```python
from build123d import *

# Parameters (mm, degrees)
SKETCH1_W           = 200
SKETCH1_H           = 100
SKETCH1_R           = 2.5
BOSS_EXTRUDE1_DEPTH = 10
FILLET1_R           = 10


with BuildPart() as part:
    # Sketch1 → Boss-Extrude1 (new body)
    with BuildSketch(Plane.XY):
        Rectangle(SKETCH1_W, SKETCH1_H)
        with Locations((90, 20)):
            Circle(SKETCH1_R, mode=Mode.SUBTRACT)
        with Locations(Location((-90, 20, 0), (0, 0, 180))):
            Circle(SKETCH1_R, mode=Mode.SUBTRACT)
        with Locations(Location((90, -20, 0), (0, 0, 180))):
            Circle(SKETCH1_R, mode=Mode.SUBTRACT)
        with Locations((-90, -20)):
            Circle(SKETCH1_R, mode=Mode.SUBTRACT)
    extrude(amount=BOSS_EXTRUDE1_DEPTH)

    # Fillet1
    fillet1_edges = [part.edges().sort_by_distance(p)[0] for p in [
        (100, -50, 5),
        (-100, -50, 5),
        (-100, 50, 5),
        (100, 50, 5),
    ]]
    fillet(fillet1_edges, radius=FILLET1_R)


solid = part.part
```
The listing builds one solid part. Answer for the finished solid, in the listing's coordinates (mm). Give positions to 0.01 mm unless a question says otherwise; leave off trailing zeros. Write each loop counter-clockwise with the first axis right and the second up, starting at its lowest first coordinate (ties: lowest second). Pieces come first, ordered by that corner, then holes. Notation, with made-up numbers: M 54,55 L 98,55 A17 cw 98,65 Z; hole C -35.75,72 d1. An arc over 180 degrees is marked long. Write each question's results on one line, items separated by ' | '.
Q1. Consider L1, parallel to Y at x = 90, z = 2.25; L2, parallel to X at y = 21.5, z = 2.75. Determine where each line is inside the solid, lowest interval first. Write a range as from..to.
Output values:
L1: -50..-22.5, -17.5..17.5, 22.5..50 | L2: -100..-92, -88..88, 92..100
Q2. A flat-ended cylindrical pin translates along its axis: P1, Ø4, axis at x = -90, y = 20, coming from the -Z side. Find the tip coordinate at first contact, or state that the pin passes through.
Output values:
P1: through
Q3. For a pull along Y with two mould halves and no side action, classify faces 1 (the cylindrical face through (96.99, 47.15, 5.07)), 2 (the cylindrical face through (91.84, -21.69, 4.93)), 3 (the flat face through (-1, 1, 10)), 4 (the cylindrical face through (96.99, -47.15, 5.07)) as released by +Y, released by -Y, zero draft, split by the parting line, or undercut.
Output values:
face 1: released by +Y | face 2: undercut | face 3: zero draft | face 4: released by -Y
Q4. Section A-A, the plane y = -20 is taken. Write down the section's boundary in (x, z).
Output values:
outline: M -100,0 L -92.5,0 L -92.5,10 L -100,10 Z; M -87.5,0 L 87.5,0 L 87.5,10 L -87.5,10 Z; M 92.5,0 L 100,0 L 100,10 L 92.5,10 Z
